from build123d import *

# Parameters (mm, degrees)
F1_W     = 20
F1_H     = 3
F2_DEPTH = 3


with BuildPart() as f2:
    # F1 (on Right) → F2 (new body)
    with BuildSketch(Plane.YZ):
        Polygon((-20, -20), (20, -20), (20, 20), (10, 20), (10, 17), (-10, 17), (-10, 20), (-20, 20), align=None)
        with Locations((0, -1.5)):
            Rectangle(F1_W, F1_H, mode=Mode.SUBTRACT)
    extrude(amount=-F2_DEPTH)


solid = f2.part
Geometry check sheet. Reference: the model listing, model coordinates, mm. A direction names the side the tool comes from. Round coordinates to 2 decimals unless told otherwise and drop trailing zeros. Loops run counter-clockwise (first coordinate to the right, second up) from the corner with the lowest first, then second, coordinate; pieces in that order, holes last. Notation, with made-up numbers: (37, 2.5) - (55, 2.5) arc R17 ccw to (55, 26.5) - close; hole circle Ø9 at (-37, 48). An arc over 180 degrees is marked (long way). Answer as CSV lines item,"result".
(1) Material ranges on line 1 along Z through (x, y) = (-1.6, -7.5); line 2 along Y through (x, z) = (-0.8, 18), recorded low to high.
Output values:
line 1,"z = -20 to -3, 0 to 17"
line 2,"y = -20 to -10, 10 to 20"
(2) Cross-section at B-B, the plane x = -1.35. Enter the section's corners in (y, z), and give its area (3 significant figures).
Output values:
outline,"(-20, -20) - (20, -20) - (20, 20) - (10, 20) - (10, 17) - (-10, 17) - (-10, 20) - (-20, 20) - close; hole (-10, -3) - (10, -3) - (10, 0) - (-10, 0) - close"
area,"1,480 mm²"
(3) Cross-section at A-A, the plane y = -8.5. Enter the section's corners in (x, z), and give its area (3 significant figures).
Output values:
outline,"(-3, -20) - (0, -20) - (0, -3) - (-3, -3) - close; (-3, 0) - (0, 0) - (0, 17) - (-3, 17) - close"
area,"102 mm²"
(4) Set-up check for faces 1 (the face through (-3, -0.3, 0.3)), 2 (the face through (-1, -10, 18)), 3 (the face through (-1, 10, -2)): record each of +Z, -Z, +X, -X, +Y, -Y from which the full face is reachable in a straight line by a thin tool's end or side.
Output values:
face 1,"+Z, -Z, -X, +Y, -Y"
face 2,"+Z, +X, -X"
face 3,"+X, -X"
(5) Release check for a two-part mould opening along Z. For faces 4 (the face through (-1, 0, -20)), 5 (the face through (-1, 0, -3)), 6 (the face through (-1, 0, 0)), 7 (the face through (-1, 10, 19)) record: released by +Z, released by -Z, zero draft, split by the parting line, or undercut.
Output values:
face 4,"released by -Z"
face 5,"undercut"
face 6,"undercut"
face 7,"zero draft"
(6) Depth check by flat-ended pin: pin 1 Ø1.5 at (x, y) = (-1, 5) entering from +Z. Enter the tip coordinate at first touch or a pass-through.
Output values:
pin 1,"stops at z = 17"
